The listing builds one solid part. Answer for the finished solid, in the listing's coordinates (mm). A direction names the side the tool comes from. Give positions to 0.01 mm unless a question says otherwise; leave off trailing zeros. Order: outer loops, then holes, each group sorted by start corner. A loop starts at its lowest first (then second) coordinate and runs counter-clockwise, first axis right, second up. Notation, with made-up numbers: (25.5, 63.5) - (63.5, 63.5) arc R21 cw to (63.5, 89.5) - close; hole circle Ø7 at (18.5, -34.75). An arc over 180 degrees is marked (long way). Answer in a Markdown table with one row per item.
from build123d import *

# Parameters (mm, degrees)
BOSS_EXTRUDE1_DEPTH                 = 184.15
SKETCH2_W                           = 63.5
SKETCH2_H                           = 95.25
CUT_EXTRUDE1_DEPTH                  = 201.603726286
F_3_8_0_375_CLEARANCE_DOWEL_HOLE1_D = 9.525
SKETCH6_W                           = 25.4
SKETCH6_H                           = 19.05
CUT_EXTRUDE2_DEPTH                  = 214.363779728
F_1_2_0_5_DIAMETER_HOLE1_D          = 12.7
FILLET1_R                           = 6.35
F_3_8_0_375_CLAMP_ADJUST_HOLE_D     = 9.525
F_3_8_0_375_CLAMP_ADJUST_HOLE_DEPTH = 82.55
F_3_8_0_375_CLAMP_ADJUST_HOLE_TIP   = 2.861598698


with BuildPart() as part:
    # Sketch1 → Boss-Extrude1 (new body)
    with BuildSketch(Plane(origin=(0, 0, 0), x_dir=(1, 0, 0), z_dir=(0, 1, 0))):
        Polygon((-38.1, 76.2), (-38.1, 0), (0, 0), (38.1, 0), (38.1, 76.2), (31.75, 76.2), (31.75, 6.35), (-31.75, 6.35), (-31.75, 76.2), align=None)
    extrude(amount=BOSS_EXTRUDE1_DEPTH)

    # Sketch2 → Cut-Extrude1 (cut, through all)
    with BuildSketch(Plane(origin=(0, 0, -6.35), x_dir=(-1, 0, 0), z_dir=(0, 0, -1))):
        with Locations((0, 47.625)):
            Rectangle(SKETCH2_W, SKETCH2_H)
    extrude(amount=-CUT_EXTRUDE1_DEPTH, mode=Mode.SUBTRACT)

    # 3/8 (0.375) Clearance Dowel Hole1 (through all)
    with Locations(Plane(origin=(38.1, 0, 0), x_dir=(0, 0, -1), z_dir=(1, 0, 0))):
        with Locations((65.0875, 19.05), (12.7, 19.05), (65.0875, 114.3)):
            Hole(F_3_8_0_375_CLEARANCE_DOWEL_HOLE1_D / 2)

    # Sketch6 → Cut-Extrude2 (cut, through all)
    with BuildSketch(Plane(origin=(38.1, 0, 0), x_dir=(0, 0, -1), z_dir=(1, 0, 0))):
        with Locations((63.5, 174.625)):
            Rectangle(SKETCH6_W, SKETCH6_H)
    extrude(amount=-CUT_EXTRUDE2_DEPTH, mode=Mode.SUBTRACT)

    # 1/2 (0.5) Diameter Hole1 (through all)
    with Locations(Plane(origin=(38.1, 0, 0), x_dir=(0, 0, -1), z_dir=(1, 0, 0))):
        with Locations((25.4, 168.275)):
            Hole(F_1_2_0_5_DIAMETER_HOLE1_D / 2)

    # Fillet1
    fillet1_edges = [part.edges().sort_by_distance(p)[0] for p in [
        (-31.75, 95.25, -3.175),
        (31.75, 95.25, -3.175),
        (34.925, 165.1, -50.8),
        (-34.925, 165.1, -50.8),
    ]]
    fillet(fillet1_edges, radius=FILLET1_R)

    # 3/8 (0.375) Clamp Adjust Hole
    with Locations(Plane(origin=(38.1, 0, 0), x_dir=(0, 0, -1), z_dir=(1, 0, 0))):
        with Locations((11.1125, 80.9752), (65.0875, 80.9752)):
            Hole(F_3_8_0_375_CLAMP_ADJUST_HOLE_D / 2, depth=F_3_8_0_375_CLAMP_ADJUST_HOLE_DEPTH)
            with Locations((0, 0, -(F_3_8_0_375_CLAMP_ADJUST_HOLE_DEPTH + F_3_8_0_375_CLAMP_ADJUST_HOLE_TIP / 2))):  # 118° drill point
                Cone(0, F_3_8_0_375_CLAMP_ADJUST_HOLE_D / 2, F_3_8_0_375_CLAMP_ADJUST_HOLE_TIP, mode=Mode.SUBTRACT)


solid = part.part
Item 1: Find section A-A on z = -42. Write down the section's boundary in (x, y).
Answer block:
| item | result |
|---|---|
| outline | (-38.1, 0) - (-31.75, 0) - (-31.75, 184.15) - (-38.1, 184.15) - close; (31.75, 0) - (38.1, 0) - (38.1, 184.15) - (31.75, 184.15) - close |
Item 2: Determine the mould class of faces 1 (the face through (-35, 178, -50.8)), 2 (the face through (34.881, 20.481, -60.545)), 3 (the face through (38.1, 91, -38)), 4 (the face through (-34.969, 76.326, -12.145)) for opening direction Z: pulls with the +Z half, pulls with the -Z half, needs draft (parallel to the pull), parting line crosses it, or undercut.
Answer block:
| item | result |
|---|---|
| face 1 | pulls with the -Z half |
| face 2 | undercut |
| face 3 | needs draft |
| face 4 | undercut |
Item 3: Find section D-D on y = 61. Write down the section's boundary in (x, z), then the cut area to 3 significant figures.
Answer block:
| item | result |
|---|---|
| outline | (-38.1, -76.2) - (-31.75, -76.2) - (-31.75, 0) - (-38.1, 0) - close; (31.75, -76.2) - (38.1, -76.2) - (38.1, 0) - (31.75, 0) - close |
| area | 968 mm² |
Item 4: Find section C-C on z = -25.4. Write down the section's boundary in (x, y) (3 decimals), then the cut area to 3 significant figures.
Answer block:
| item | result |
|---|---|
| outline | (-38.1, 0) - (-31.75, 0) - (-31.75, 161.925) - (-38.1, 161.925) - close; (-38.1, 174.625) - (-31.75, 174.625) - (-31.75, 184.15) - (-38.1, 184.15) - close; (31.75, 0) - (38.1, 0) - (38.1, 161.925) - (31.75, 161.925) - close; (31.75, 174.625) - (38.1, 174.625) - (38.1, 184.15) - (31.75, 184.15) - close |
| area | 2,180 mm² |
Item 5: Which of the six approach directions +Z, -Z, +X, -X, +Y, -Y give full straight-line access (tool end or side, diameter ignored) to faces 5 (the face through (-35, 165.1, -67)), 6 (the face through (0, 136, -6.35)), 7 (the face through (-29.94, 93.34, -3.13))?
Answer block:
| item | result |
|---|---|
| face 5 | -Z, +X, -X, +Y |
| face 6 | -Z, +Y, -Y |
| face 7 | +Z, -Z, -Y |
Item 6: Find section B-B on y = 114.3. Write down the section's boundary in (x, z) (3 decimals), then the cut area to 3 significant figures.
Answer block:
| item | result |
|---|---|
| outline | (-38.1, -76.2) - (-31.75, -76.2) - (-31.75, -69.85) - (-38.1, -69.85) - close; (-38.1, -60.325) - (-31.75, -60.325) - (-31.75, -6.35) - (31.75, -6.35) - (31.75, -60.325) - (38.1, -60.325) - (38.1, 0) - (-38.1, 0) - close; (31.75, -76.2) - (38.1, -76.2) - (38.1, -69.85) - (31.75, -69.85) - close |
| area | 1,250 mm² |
Item 7: Each of these flat-tipped pins is pushed along its axis until it touches: P1, Ø7.5, axis at y = 114.3, z = -65.09, coming from the +X side; P2, Ø5, axis at x = -35, z = -67, coming from the +Y side; P3, Ø7, axis at x = -33.5, y = 177, coming from the -Z side. Where does it stop, or does it pass through?
Answer block:
| item | result |
|---|---|
| P1 | through |
| P2 | y = 165.1 |
| P3 | z = -50.8 |
Item 8: Consider line 1 (X direction, y = 48, z = -58.5); line 2 (Y direction, x = -33, z = -25); line 3 (Z direction, x = -14, y = 111). Determine where each line is inside the solid, lowest interval first.
Answer block:
| item | result |
|---|---|
| line 1 | -38.1 to -31.75, 31.75 to 38.1 |
| line 2 | 0 to 161.94, 174.61 to 184.15 |
| line 3 | -6.35 to 0 |
